Read the model definition and answer for the solid it produces. Units are mm, in the model's axes. Coordinates: 2 decimals unless noted, no trailing zeros. Write each loop counter-clockwise with the first axis right and the second up, starting at its lowest first coordinate (ties: lowest second). Pieces come first, ordered by that corner, then holes. Notation, with made-up numbers: (72.25, 68.5) -> (122.25, 68.5) arc R12 ccw to (122.25, 89.5) -> close; hole circle Ø4 at (72, 42.5). An arc over 180 degrees is marked (long way). One line per item, written item: value. Start each with the question number.
1. Consider line 1 along X through (y, z) = (256, 3498); line 2 along Y through (x, z) = (-42.5, 3507.25); line 3 along Y through (x, z) = (-452.5, 3502.5) (3 decimals). Determine where each line is inside the solid, lowest interval first.
2. Given P1, Ø1.5, axis at x = -110.5, z = 3508, coming from the +Y side; P2, Ø8, axis at x = 689, z = 3509.5, coming from the -Y side; P3, Ø1, axis at y = -142.5, z = 3514.5, coming from the +X side, each flat-ended and moving along its own axis, determine where each tip first touches the part or whether it passes through.
3. Find section B-B, the plane y = -400. Write down the section's boundary in (x, z), and give its area (3 significant figures).
4. Find section C-C, the plane z = 3516.5. Write down the section's boundary in (x, y) (3 decimals).
5. Find section A-A, the plane x = -117. Write down the section's boundary in (y, z).
6. Find section D-D, the plane y = -788. Write down the section's boundary in (x, z), and give its area (3 significant figures).
Solid Edge part; units mm, degrees
sketch "Sketch1" plane through (0, 0, 0) normal (0, -1, 0) x (1, 0, 0)
  line L0 (-647.7, 0) -> (-647.7, 3349.6026)
  line L1 (0, 0) -> (0, 3810)
  line L2 (0, 0) -> (-647.7, 0)
  arc A0 (-647.7, 3349.6026) -> (0, 3810) centre (0, 3124.2) cw
revolve "RevolvedProtrusion1" add sketch "Sketch1" angle 360 about axis through (0, 0, 0) along (0, 0, 1)
sketch "Sketch2" plane through (0, 0, 3496.7418) normal (0, 0, 1) x (1, 0, 0)
  arc A0 (1113.6113, 339.3453) -> (-699.7577, -930.3894) centre (-700.215, 1000.0106) cw
  line L0 (-699.7577, -930.3894) -> (-699.7577, 441.2108)
  arc A1 (-175.2713, 808.4602) -> (-699.7577, 441.2108) centre (-700.2149, 1000.0106) cw
  line L1 (-175.2713, 808.4602) -> (1113.6113, 339.3453)
extrude "ExtrudedProtrusion_2" add sketch "Sketch2" along normal blind 25.4
sketch "Sketch3" plane through (0, 0, 0) normal (0, -1, 0) x (1, 0, 0)
  line L0 (-647.7, 0) -> (-647.7, 3349.6026)
  line L1 (0, 0) -> (0, 3810)
  line L2 (0, 0) -> (-647.7, 0)
  arc A0 (-647.7, 3349.6026) -> (0, 3810) centre (0, 3124.2) cw
revolve "RevolvedCutout1" cut sketch "Sketch3" angle 360 about axis through (0, 0, 0) along (0, 0, 1)
Answer block:
1. line 1: x = -699.76 to -514.84, 514.84 to 1081.05
1. line 2: y = -814.89 to -567.26, 567.26 to 760.14
1. line 3: y = -914.43 to -349.935, 349.935 to 499.117
2. P1: stops at y = 785.16
2. P2: stops at y = -344.47
2. P3: stops at x = 856.14
3. outline: (-699.76, 3496.74) -> (-414.17, 3496.74) arc R557.07 cw to (-389.83, 3522.14) -> (-699.76, 3522.14) -> close; (389.83, 3522.14) arc R557.07 cw to (414.17, 3496.74) -> (628.85, 3496.74) -> (628.85, 3522.14) -> close
3. area: 13,300 mm2
4. outline: (-699.758, -930.389) arc R1930.4 ccw to (1113.611, 339.345) -> (-175.271, 808.46) arc R558.8 cw to (-699.758, 441.211) -> close; hole circle Ø1125.029 at (0, 0)
5. outline: (-840.18, 3496.74) -> (-563.78, 3496.74) arc R675.75 cw to (-546.15, 3522.14) -> (-840.18, 3522.14) -> close; (546.15, 3522.14) arc R675.75 cw to (563.78, 3496.74) -> (787.25, 3496.74) -> (787.25, 3522.14) -> close
6. outline: (-699.76, 3496.74) -> (27.43, 3496.74) -> (27.43, 3522.14) -> (-699.76, 3522.14) -> close
6. area: 18,500 mm2
